Autodesk Inventor part; units mm, degrees
ref_plane "Work Plane1" through (6.35, -34.925, 15.875) normal (0, 0, 1) x (1, 0, 0)
ref_plane "YZ Plane" through (0, 0, 0) normal (1, 0, 0) x (0, 1, 0)
ref_plane "XZ Plane" through (0, 0, 0) normal (0, 1, 0) x (-1, 0, 0)
ref_plane "Work Plane1" through (6.35, -34.925, 15.875) normal (0, 0, 1) x (1, 0, 0)
sketch "Sketch3" plane through (6.35, -34.925, 15.875) normal (0, 0, 1) x (1, 0, 0)
  line L0 (1.5875, 69.85) -> (1.5875, 0)
  line L1 (14.2875, 0) -> (1.5875, 34.925) construction
  line L2 (1.5875, 34.925) -> (14.2875, 69.85) construction
  spline S0 degree 2 poles (14.2875, 0) (1.5875, 34.925) (14.2875, 69.85) knots 1 1 1 2 2 2
  line L3 (1.5875, 69.85) -> (14.2875, 69.85)
  line L4 (14.2875, 0) -> (1.5875, 0)
  point P0 (-6.35, 34.925)
  dimension "d9" = 12.7
  dimension "d10" = 12.7
extrude "Extrusion3" add sketch "Sketch3" against normal blind 31.75
sketch "Sketch4" plane through (7.9375, -34.925, 15.875) normal (-1, 0, 0) x (0, 0, 1)
  line L0 (0, 69.85) -> (0, 0)
  line L1 (0, 69.85) -> (-31.75, 69.85)
  line L2 (-31.75, 0) -> (-31.75, 69.85)
  line L3 (0, 0) -> (-31.75, 0)
  line L4 (0, 0) -> (-31.75, 0) construction
  line L5 (-15.875, 0) -> (-15.875, 69.85) construction
  line L6 (0, 69.85) -> (-31.75, 69.85) construction
  circle A0 centre (-15.875, 33.02) radius 0.635
  circle A1 centre (-15.875, 36.83) radius 0.635
  circle A2 centre (-15.875, 34.925) radius 3.6195
  circle A3 centre (-15.875, 52.07) radius 0.635
  circle A4 centre (-15.875, 55.88) radius 0.635
  circle A5 centre (-15.875, 53.975) radius 3.6195
  circle A6 centre (-15.875, 13.97) radius 0.635
  circle A7 centre (-15.875, 17.78) radius 0.635
  circle A8 centre (-15.875, 15.875) radius 3.6195
  circle A9 centre (-15.875, 33.02) radius 0.635
  circle A10 centre (-15.875, 36.83) radius 0.635
  circle A11 centre (-15.875, 34.925) radius 3.6195
  dimension "d13" = 1.27
  dimension "d14" = 1.27
  dimension "d15" = 1.905
  dimension "d16" = 1.905
  dimension "d17" = 7.239
  dimension "d20" = 19.05
  dimension "d23" = 19.05
extrude "Extrusion4" add sketch "Sketch4" against normal blind 9.017 contours A2 | A5 | A8
sketch "Sketch5" plane through (16.9545, -34.925, 15.875) normal (1, 0, 0) x (0, 0, -1)
  arc A0 (15.3692, 57.559) -> (16.3808, 57.559) centre (15.875, 53.975) ccw
  circle A1 centre (15.875, 55.88) radius 0.635
  circle A2 centre (15.875, 52.07) radius 0.635
  circle A3 centre (15.875, 34.925) radius 3.6195
  circle A4 centre (15.875, 33.02) radius 0.635
  circle A5 centre (15.875, 36.83) radius 0.635
  arc A6 (16.3808, 12.291) -> (15.3692, 12.291) centre (15.875, 15.875) ccw
  circle A7 centre (15.875, 17.78) radius 0.635
  circle A8 centre (15.875, 13.97) radius 0.635
extrude "Extrusion5" cut sketch "Sketch5" against normal blind 9.017 contours A1 | A2 | A4 | A5 | A7 | A8
properties part number "LED Reflector"
Here's how the part is built. I have some questions about the finished solid (model axes, mm). A direction names the side the tool comes from. Give positions to 0.01 mm unless a question says otherwise; leave off trailing zeros. Answer as a JSON object with one key per item and string values. Group by question number.
Item 1: Which directions (+Z, -Z, +X, -X, +Y, -Y) give clear straight access to the entire face, cutting with the end or side of a thin tool? Please do faces 1 (the flat face through (13, 0, 15.875)), 2 (the flat face through (16.954, 19, 0)), 3 (the cylindrical face through (15.6, 3.59, -0.47)).
Item 2: If we mould it in two halves opening along Y, with no side actions, what happens to faces 4 (the cylindrical face through (16.389, -15.434, 0.152)), 5 (the flat face through (7.938, 0, 0)), 6 (the flat face through (14, 34.925, 0))? For each: pulls with the +Y half, pulls with the -Y half, needs draft (parallel to the pull), parting line crosses it, or undercut.
Item 3: Please list where these lines run through material, in increasing order: probe 1 along X at (y, z) = (-2.5, -13.5); probe 2 along Z at (x, y) = (16.5, 0.5); probe 3 along X at (y, z) = (-13, -11.5).
Item 4: For P1, Ø2, axis at y = -1, z = 1, coming from the +X side; P2, Ø1, axis at y = -11, z = 0, coming from the +X side; P3, Ø1, axis at x = 17, y = 3.5, coming from the -Z side, each with a flat end and sliding along its axis, tell me the tip position at first contact or that it passes through.
Result set:
{
 "1": {"face 1": "+Z, +X, -X, +Y, -Y", "face 2": "+Z, -Z, +X", "face 3": "+X"},
 "2": {"face 4": "undercut", "face 5": "needs draft", "face 6": "pulls with the +Y half"},
 "3": {"probe 1": "7.94 to 14.32", "probe 2": "-3.58 to 3.58", "probe 3": "7.94 to 15.17"},
 "4": {"P1": "x = 16.95", "P2": "x = 14.98", "P3": "z = -2.02"}
}
